Design review of the part shown in the three views and the two pictorial views. Dimensions are in mm from the part's minimum x, y and z. A direction names the side the tool comes from. Give positions to 0.01 mm unless a question says otherwise; leave off trailing zeros. Order: outer loops, then holes, each group sorted by start corner. A loop starts at its lowest first (then second) coordinate and runs counter-clockwise, first axis right, second up. Notation, with made-up numbers: (47.5, 69) - (66.5, 69) arc R23 ccw to (66.5, 102) - close; hole circle Ø10 at (5, -21.5). An arc over 180 degrees is marked (long way). Put each result on its own line as item: value. Start each with the question number.
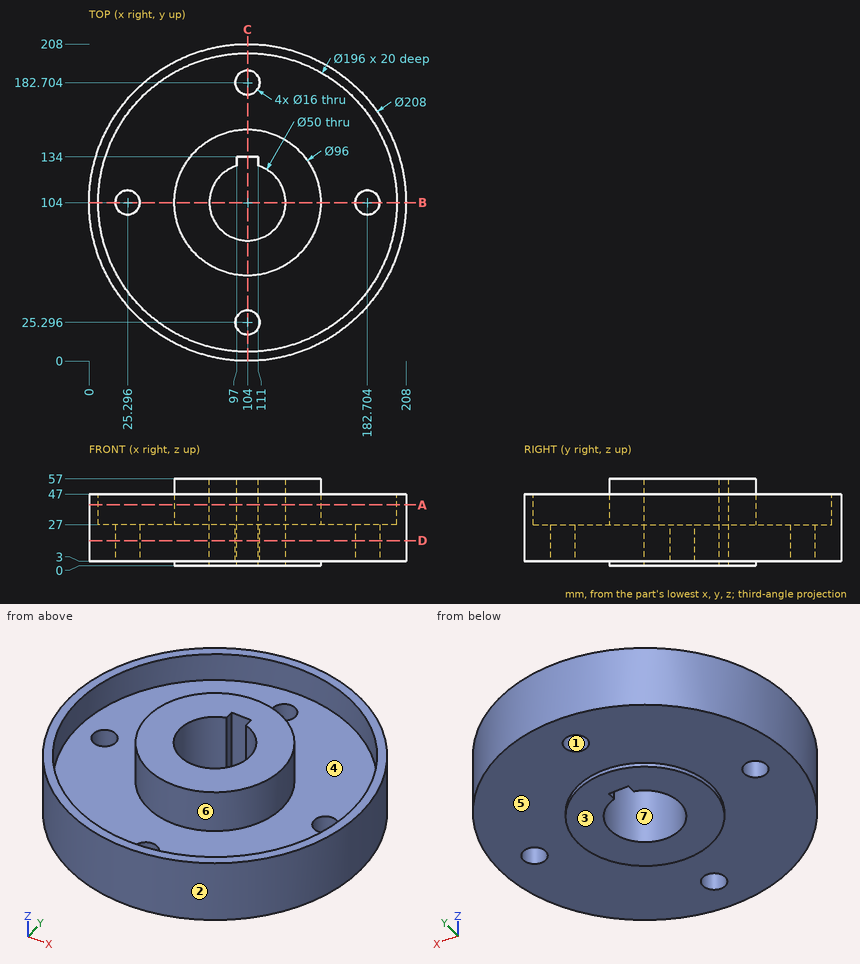
1. Add section D-D, the plane z = 16.5. Give the boundary of the cut face in (x, y) (1 decimal).
2. Clearance check with flat-ended pins moving along their axes: pin 1 (5 mm diameter, centred on x = 109, z = 35, fed in from -Y); pin 2 (3 mm diameter, centred on x = 95.5, z = 7.5, fed in from +Y); pin 3 (13 mm diameter, centred on x = 104, y = 25.3, fed in from -Z); pin 4 (10 mm diameter, centred on y = 128.5, z = 46, fed in from -X) (1 decimal). State where each tip first meets the part, or that it passes through.
3. Add section C-C, the plane x = 104. Give the boundary of the cut face in (y, z) (1 decimal), then the cut area to 3 significant figures.
4. The part is to be moulded in two halves that separate along Y. For the marked faces 1, 2, 3 and 4, say which applies: released by +Y, released by -Y, zero draft, split by the parting line, or undercut.
5. Add section A-A, the plane z = 40. Give the boundary of the cut face in (x, y), then the cut area to 3 significant figures.
6. Tool access review of the marked faces 5, 6 and 7: name each direction out of +Z, -Z, +X, -X, +Y, -Y from which nothing blocks a thin tool from reaching the whole face with its end or side.
7. Add section B-B, the plane y = 104. Give the boundary of the cut face in (x, z) (1 decimal).
8. Wall thickness on line 1 (Y direction, x = 105.5, z = 37.5) (1 decimal); line 2 (Y direction, x = 104, z = 12.5) (1 decimal); line 3 (X direction, y = 110, z = 16.5) (1 decimal): over which ranges is each line inside the solid? List them lowest first. Write a range as from..to.
Found:
1. outline: circle Ø208 at (104, 104); hole circle Ø16 at (25.3, 104); hole circle Ø16 at (104, 25.3); hole circle Ø16 at (104, 182.7); hole (97, 128) arc R25 ccw (long way) to (111, 128) - (111, 134) - (97, 134) - close; hole circle Ø16 at (182.7, 104)
2. pin 1: stops at y = 0.03
2. pin 2: stops at y = 207.76
2. pin 3: passes through
2. pin 4: stops at x = 1.8
3. outline: (0, 3) - (17.3, 3) - (17.3, 27) - (6, 27) - (6, 47) - (0, 47) - close; (33.3, 3) - (56, 3) - (56, 0) - (79, 0) - (79, 57) - (56, 57) - (56, 27) - (33.3, 27) - close; (134, 0) - (152, 0) - (152, 3) - (174.7, 3) - (174.7, 27) - (152, 27) - (152, 57) - (134, 57) - close; (190.7, 3) - (208, 3) - (208, 47) - (202, 47) - (202, 27) - (190.7, 27) - close
3. area: 4,500 mm^2
4. face 1: undercut
4. face 2: split by the parting line
4. face 3: zero draft
4. face 4: undercut
5. outline: circle Ø208 at (104, 104); circle Ø96 at (104, 104); hole circle Ø196 at (104, 104); hole (97, 128) arc R25 ccw (long way) to (111, 128) - (111, 134) - (97, 134) - close
5. area: 9,010 mm^2
6. face 5: -Z
6. face 6: +Z
6. face 7: +Z, -Z
7. outline: (0, 3) - (17.3, 3) - (17.3, 27) - (6, 27) - (6, 47) - (0, 47) - close; (33.3, 3) - (56, 3) - (56, 0) - (79, 0) - (79, 57) - (56, 57) - (56, 27) - (33.3, 27) - close; (129, 0) - (152, 0) - (152, 3) - (174.7, 3) - (174.7, 27) - (152, 27) - (152, 57) - (129, 57) - close; (190.7, 3) - (208, 3) - (208, 47) - (202, 47) - (202, 27) - (190.7, 27) - close
8. line 1: y = 0..6, 56..79, 134..152, 202..208
8. line 2: y = 0..17.3, 33.3..79, 134..174.7, 190.7..208
8. line 3: x = 0.2..20, 30.6..79.7, 128.3..177.4, 188..207.8
